```python
from build123d import *

# Parameters (mm, degrees)
SKETCH3_R   = 14.732
SKETCH3_R_2 = 6.9342


with BuildPart() as part:
    # Sketch1 → Revolve1 (revolve)
    with BuildSketch(Plane.XY, mode=Mode.PRIVATE) as revolve1_sk:
        Polygon((-34.798, -14.732), (-12.954, -14.732), (-12.954, -10.6172), (-34.798, -10.7696), align=None)
    revolve(revolve1_sk.sketch.rotate(Axis((-34.798, 0, 0), (1, 0, 0)), 270), axis=Axis((-34.798, 0, 0), (1, 0, 0)))


with BuildPart() as body_2:
    # Sketch2 → Revolve2 (revolve)
    with BuildSketch(Plane.XY, mode=Mode.PRIVATE) as revolve2_sk:
        Polygon((10.7696, 34.798), (10.6172, 12.954), (14.732, 12.954), (14.732, 34.798), align=None)
    revolve(revolve2_sk.sketch.rotate(Axis((0, 0, 0), (0, 1, 0)), 90), axis=Axis((0, 0, 0), (0, 1, 0)))


with BuildPart() as sweep1_tool:
    # Sweep1: sweep along a path in Sketch4
    with BuildLine(Plane.XY) as sweep1_path:
        ThreePointArc((-12.954, 0), (-3.794139, 3.794139), (0, 12.954))
    # Sketch3 → Sweep1 (sweep)
    with BuildSketch(Plane(origin=(-12.954, 0, 0), x_dir=(0, 0, -1), z_dir=(1, 0, 0))):
        Circle(SKETCH3_R)
        Circle(SKETCH3_R_2, mode=Mode.SUBTRACT)
    sweep(path=sweep1_path.line)


with BuildPart() as part_1:
    add(part.part)


with BuildPart() as part_2:
    # Sweep1: joined with sweep1_tool
    add(part_1.part.fuse(sweep1_tool.part, body_2.part, tol=0.00001))


solid = part_2.part
```
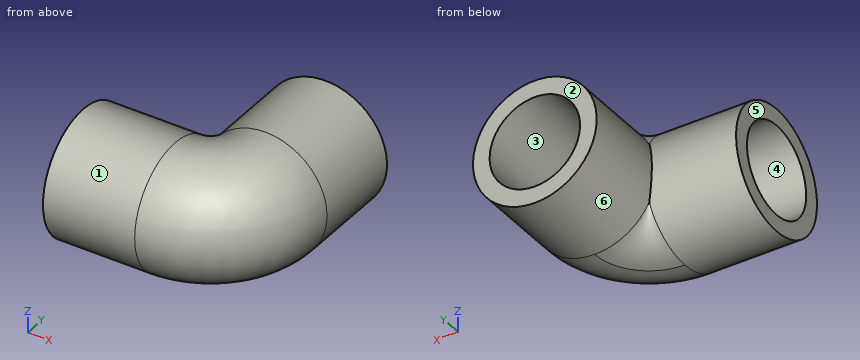
Source: CAD feature listing. Evaluate the final solid. Frame: model axes, mm. Face numbers are marked on the shaded views. A direction names the side the tool comes from. Give positions to 0.01 mm unless a question says otherwise; leave off trailing zeros. Order: outer loops, then holes, each group sorted by start corner. A loop starts at its lowest first (then second) coordinate and runs counter-clockwise, first axis right, second up.
(1) Material intervals for line 1 along Z through (x, y) = (-32, -4); line 2 along Y through (x, z) = (-19, 8.5); line 3 along Y through (x, z) = (-9.5, 3.25), sorted ascending.
(2) Section query A-A (x = -24). Return the cut outline in (y, z).
(3) Pull-direction query (Z, two-part tool) for the marked faces 4, 5 and 6; classes: +Z half, -Z half, draft (parallel to the pull), parting line (faces both ways), or undercut.
(4) Contact query for flat-ended pins moving along their axis: P1, Ø5, axis at x = -24.5, z = 6.5, coming from the +Y side; P2, Ø4, axis at x = 2.5, z = 4.5, coming from the +Y side; P3, Ø12, axis at x = -21.5, y = 28.5, coming from the -Z side; P4, Ø8, axis at x = -7.5, y = 16, coming from the -Z side. Output: stop coordinate, or through.
(5) Access query for the marked faces 1, 2 and 3. Directions: +Z, -Z, +X, -X, +Y, -Y. A direction counts if a zero-diameter tool reaches every point of the face in a straight line with its end or side. Return the directions, or none.
Outcome:
1. line 1: z = -14.18 to -9.98, 9.98 to 14.18
1. line 2: y = -12.03 to -6.43, 6.43 to 12.03
1. line 3: y = -14.15 to -5.81, 7.06 to 12.95
2. outline: circle Ø29.46 at (0, 0); hole circle Ø21.39 at (0, 0)
3. face 4: undercut
3. face 5: draft
3. face 6: parting line
4. P1: stops at y = 14.18
4. P2: stops at y = 12.95
4. P3: passes through
4. P4: stops at z = -14.31
5. face 1: -X
5. face 2: +Z, -Z, +X, -X, +Y
5. face 3: +Y
